Read the model definition and answer for the solid it produces. Units are mm, in the model's axes. Face numbers are marked on the shaded views. Coordinates: 2 decimals unless noted, no trailing zeros. Write each loop counter-clockwise with the first axis right and the second up, starting at its lowest first coordinate (ties: lowest second). Pieces come first, ordered by that corner, then holes. Notation, with made-up numbers: (-37.5, 83) -> (-25.5, 83) arc R38 cw to (-25.5, 122) -> close; hole circle Ø3 at (5.25, 4.25). An arc over 180 degrees is marked (long way). Use CSV: the item, a comma, the result in double quotes. Start each with the question number.
from build123d import *

# Parameters (mm, degrees)
SKETCH_W   = 40
SKETCH_H   = 30
SKETCH_R   = 2.65
SKETCH_R_2 = 1.65
PAD_DEPTH  = 3
FILLET_R   = 3


with BuildPart() as part:
    # Sketch → Pad (new body)
    with BuildSketch(Plane.XY):
        with Locations((10, 5)):
            Rectangle(SKETCH_W, SKETCH_H)
        Circle(SKETCH_R, mode=Mode.SUBTRACT)
        with Locations((20, 0)):
            Circle(SKETCH_R, mode=Mode.SUBTRACT)
        with Locations((-5, 15)):
            Circle(SKETCH_R_2, mode=Mode.SUBTRACT)
        with Locations((25, 15)):
            Circle(SKETCH_R_2, mode=Mode.SUBTRACT)
    extrude(amount=PAD_DEPTH)

    # Fillet
    fillet_edges = [part.edges().sort_by_distance(p)[0] for p in [
        (-10, -10, 1.5),
        (30, -10, 1.5),
        (-10, 20, 1.5),
        (30, 20, 1.5),
    ]]
    fillet(fillet_edges, radius=FILLET_R)


solid = part.part
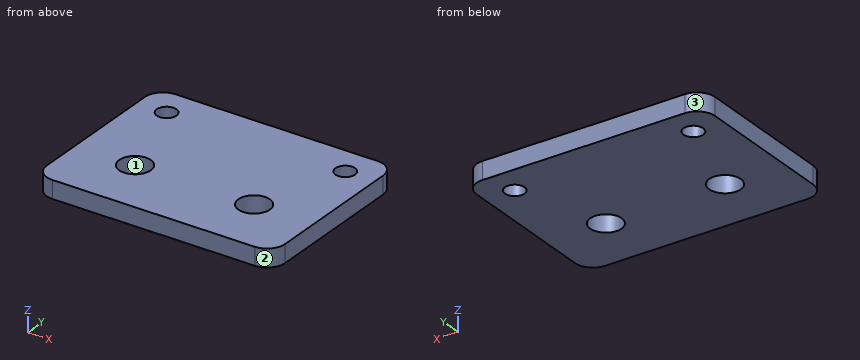
1) Section A-A, the plane x = 25 is taken. Give the vertices of the cut face in (y, z), plus the area to 3 significant figures.
2) Section C-C, the plane x = 20 is taken. Give the vertices of the cut face in (y, z), plus the area to 3 significant figures.
3) This flat-tipped pin is pushed along its axis until it touches: pin 1 (3 mm diameter, centred on x = 20, y = 0, fed in from +Z). Where does it stop, or does it pass through?
4) Find the intervals of material crossed by line 1 along Y through (x, z) = (20, 2); line 2 along X through (y, z) = (16.5, 2.4); line 3 along X through (y, z) = (-0.5, 1.5), in increasing order.
5) Section B-B, the plane z = 1.15 is taken. Give the vertices of the cut face in (x, y), plus the area to 3 significant figures.
6) The mould has two halves that part along Y. Classify the marked faces 1, 2 and 3: pulls with the +Y half, pulls with the -Y half, needs draft (parallel to the pull), parting line crosses it, or undercut.
The answers:
1,outline,"(-10, 0) -> (13.35, 0) -> (13.35, 3) -> (-10, 3) -> close; (16.65, 0) -> (20, 0) -> (20, 3) -> (16.65, 3) -> close"
1,area,"80.1 mm^2"
2,outline,"(-10, 0) -> (-2.65, 0) -> (-2.65, 3) -> (-10, 3) -> close; (2.65, 0) -> (20, 0) -> (20, 3) -> (2.65, 3) -> close"
2,area,"74.1 mm^2"
3,pin 1,"passes through"
4,line 1,"y = -10 to -2.65, 2.65 to 20"
4,line 2,"x = -10 to -5.69, -4.31 to 24.31, 25.69 to 30"
4,line 3,"x = -10 to -2.6, 2.6 to 17.4, 22.6 to 30"
5,outline,"(-10, -7) arc R3 ccw to (-7, -10) -> (27, -10) arc R3 ccw to (30, -7) -> (30, 17) arc R3 ccw to (27, 20) -> (-7, 20) arc R3 ccw to (-10, 17) -> close; hole circle Ø3.3 at (-5, 15); hole circle Ø5.3 at (0, 0); hole circle Ø5.3 at (20, 0); hole circle Ø3.3 at (25, 15)"
5,area,"1,130 mm^2"
6,face 1,"undercut"
6,face 2,"pulls with the -Y half"
6,face 3,"pulls with the +Y half"
